from build123d import *

# Parameters (mm, degrees)
F0_R     = 3
F1_DEPTH = 30
F2_SIZE  = 0.7
F4_DEPTH = 31


with BuildPart() as f1:
    # F0 (on Right) → F1 (new body)
    with BuildSketch(Plane.YZ):
        Circle(F0_R)
    extrude(amount=F1_DEPTH)

    # F2
    f2_edges = [f1.edges().sort_by_distance(p)[0] for p in [
        (30, -3, 0),
        (0, -3, 0),
    ]]
    chamfer(f2_edges, length=F2_SIZE)

    # F3 (on face) → F4 (cut)
    with BuildSketch(Plane.YZ.offset(30)):
        with BuildLine():
            Line((-3.31023, -1), (-2.219542, -0.603022))
            ThreePointArc((-2.219542, -0.603022), (-2.3, 0), (-2.219542, 0.603022))
            Line((-2.219542, 0.603022), (-3.31023, 1))
            Line((-3.31023, 1), (-3.31023, -1))
        make_face()
        with BuildLine():
            Line((-2.219542, -0.603022), (-1.936492, -0.5))
            ThreePointArc((-1.936492, -0.5), (2, 0), (-1.936492, 0.5))
            Line((-1.936492, 0.5), (-2.219542, 0.603022))
            ThreePointArc((-2.219542, 0.603022), (-2.3, 0), (-2.219542, -0.603022))
        make_face()
    extrude(amount=-F4_DEPTH, mode=Mode.SUBTRACT)


solid = f1.part
Work out the finished part from the listing and answer in its coordinate system (mm). Round coordinates to 2 decimals unless told otherwise and drop trailing zeros. Write each loop counter-clockwise with the first axis right and the second up, starting at its lowest first coordinate (ties: lowest second). Pieces come first, ordered by that corner, then holes. Notation, with made-up numbers: (-2, 61) -> (12, 61) arc R25 ccw to (12, 82) -> close; hole circle Ø5 at (3.25, -10.75). An arc over 180 degrees is marked (long way). Write each question's results on one line, items separated by ' | '.
Item 1: Find the intervals of material crossed by line 1 along Z through (x, y) = (6.5, 0); line 2 along Y through (x, z) = (11.75, 0); line 3 along Z through (x, y) = (26, -1.3), in increasing order. Write a range as [from, to].
Result set:
line 1: [-3, -2], [2, 3] | line 2: [2, 3] | line 3: [-2.7, -1.52], [1.52, 2.7]
Item 2: A cutting plane is placed at C-C, the plane x = 12. Determine the outline of the cut face in (y, z).
Result set:
outline: (-2.88, -0.84) arc R3 ccw (long way) to (-2.88, 0.84) -> (-2.22, 0.6) -> (-1.94, 0.5) arc R2 cw (long way) to (-1.94, -0.5) -> (-2.22, -0.6) -> close
Item 3: A cutting plane is placed at B-B, the plane z = 0. Determine the outline of the cut face in (x, y), plus the area to 3 significant figures.
Result set:
outline: (0, 2) -> (30, 2) -> (30, 2.3) -> (29.3, 3) -> (0.7, 3) -> (0, 2.3) -> close | area: 29.5 mm^2
Item 4: Flat-ended cylindrical pins translate along their axes: P1, Ø1, axis at x = 9.5, z = -1.5, coming from the +Y side; P2, Ø2, axis at x = 24, z = 1.5, coming from the +Y side. Find the tip coordinate at first contact, or state that the pin passes through.
Result set:
P1: y = 2.83 | P2: y = 2.96
Item 5: A cutting plane is placed at A-A, the plane y = 0. Determine the outline of the cut face in (x, z).
Result set:
outline: (0, -2.3) -> (0.7, -3) -> (29.3, -3) -> (30, -2.3) -> (30, -2) -> (0, -2) -> close; (0, 2) -> (30, 2) -> (30, 2.3) -> (29.3, 3) -> (0.7, 3) -> (0, 2.3) -> close
